Geometry check sheet. Reference: the model listing, model coordinates, mm. A direction names the side the tool comes from. Round coordinates to 2 decimals unless told otherwise and drop trailing zeros. Write each loop counter-clockwise with the first axis right and the second up, starting at its lowest first coordinate (ties: lowest second). Pieces come first, ordered by that corner, then holes. Notation, with made-up numbers: M 33,13.25 L 47,13.25 A21 cw 47,47.25 Z; hole C 20,76.5 d7. An arc over 180 degrees is marked long. Use a Markdown table: item, result.
```python
from build123d import *

# Parameters (mm, degrees)
SKETCH1_R               = 1.5
BOSS_EXTRUDE1_DEPTH     = 3.175
CUT_EXTRUDE1_DEPTH      = 131.960225355
CUT_EXTRUDE1_DEPTH_BACK = 131.960225355
SKETCH2_R               = 1.5
CUT_EXTRUDE2_DEPTH      = 131.960225355
CUT_EXTRUDE2_DEPTH_BACK = 131.960225355
SKETCH3_R               = 1.5
CUT_EXTRUDE4_DEPTH      = 40
SKETCH6_R               = 1.6
CUT_EXTRUDE5_DEPTH      = 10


with BuildPart() as part:
    # Sketch1 → Boss-Extrude1 (new body)
    with BuildSketch(Plane(origin=(0, 0, 0), x_dir=(1, 0, 0), z_dir=(0, 1, 0))):
        with BuildLine():
            Line((-10.5, 0), (-10.5, -120))
            ThreePointArc((-10.5, -120), (0, -130.5), (10.5, -120))
            Line((10.5, -120), (10.5, 0))
            ThreePointArc((10.5, 0), (0, 10.5), (-10.5, 0))
        make_face()
        with Locations(Location((0, 0, 0), (0, 0, 270))):
            Circle(SKETCH1_R, mode=Mode.SUBTRACT)
        with Locations(Location((0, -120, 0), (0, 0, 270))):
            Circle(SKETCH1_R, mode=Mode.SUBTRACT)
    extrude(amount=BOSS_EXTRUDE1_DEPTH)

    # Sketch2 → Cut-Extrude1 (cut, two sides: drawn at the far end of the back side and taken through both)
    with BuildSketch(Plane.XZ.offset(-CUT_EXTRUDE1_DEPTH_BACK)):
        with Locations(Location((0, 20, 0), (0, 0, 270))):
            Circle(SKETCH2_R)
    extrude(amount=CUT_EXTRUDE1_DEPTH + CUT_EXTRUDE1_DEPTH_BACK, mode=Mode.SUBTRACT)

    # Sketch3 → Cut-Extrude2 (cut, two sides: drawn at the far end of the back side and taken through both)
    with BuildSketch(Plane(origin=(0, 3.175, 0), x_dir=(1, 0, 0), z_dir=(0, 1, 0)).offset(-CUT_EXTRUDE2_DEPTH_BACK)):
        with Locations(Location((0, -100, 0), (0, 0, 270))):
            Circle(SKETCH3_R)
    extrude(amount=CUT_EXTRUDE2_DEPTH + CUT_EXTRUDE2_DEPTH_BACK, mode=Mode.SUBTRACT)

    # Sketch5 → Cut-Extrude4 (cut)
    with BuildSketch(Plane.XZ):
        with BuildLine():
            Line((-8.5, 10), (-8.5, 50))
            ThreePointArc((-8.5, 50), (-7.5, 51), (-6.5, 50))
            Line((-6.5, 50), (-6.5, 10))
            ThreePointArc((-6.5, 10), (-7.5, 9), (-8.5, 10))
        make_face()
        with BuildLine():
            Line((6.5, 50), (6.5, 10))
            ThreePointArc((6.5, 10), (7.5, 9), (8.5, 10))
            Line((8.5, 10), (8.5, 50))
            ThreePointArc((8.5, 50), (7.5, 51), (6.5, 50))
        make_face()
        with BuildLine():
            Line((8.5, 110), (8.5, 70))
            ThreePointArc((8.5, 70), (7.5, 69), (6.5, 70))
            Line((6.5, 70), (6.5, 110))
            ThreePointArc((6.5, 110), (7.5, 111), (8.5, 110))
        make_face()
        with BuildLine():
            Line((-6.5, 70), (-6.5, 110))
            ThreePointArc((-6.5, 110), (-7.5, 111), (-8.5, 110))
            Line((-8.5, 110), (-8.5, 70))
            ThreePointArc((-8.5, 70), (-7.5, 69), (-6.5, 70))
        make_face()
    extrude(amount=-CUT_EXTRUDE4_DEPTH, mode=Mode.SUBTRACT)

    # Sketch6 → Cut-Extrude5 (cut)
    with BuildSketch(Plane.XZ):
        with Locations(Location((0, 70.85, 0), (0, 0, 270))):
            Circle(SKETCH6_R)
        with Locations(Location((0, 32.85, 0), (0, 0, 270))):
            Circle(SKETCH6_R)
    extrude(amount=-CUT_EXTRUDE5_DEPTH, mode=Mode.SUBTRACT)


solid = part.part
```
Item 1: Cross-section at B-B, the plane y = 2. Count the separate pieces of the cut face and the enclosed holes in it, and give its area (3 significant figures).
Outcome:
| item | result |
|---|---|
| separate pieces | 1 |
| enclosed holes | 10 |
| area | 2,490 mm2 |
Item 2: Go/stop test with a flat-tipped pin: pin 1 (1 mm diameter, centred on x = -7.5, y = 2.5, fed in from +Z). Record where the tip stops, or that it passes through.
Outcome:
| item | result |
|---|---|
| pin 1 | stops at z = 127.83 |
Item 3: Cross-section at C-C, the plane z = 77.5. Record the cut outline in (x, y) (3 decimals), and give its area (3 significant figures).
Outcome:
| item | result |
|---|---|
| outline | M -10.5,0 L -8.5,0 L -8.5,3.175 L -10.5,3.175 Z; M -6.5,0 L 6.5,0 L 6.5,3.175 L -6.5,3.175 Z; M 8.5,0 L 10.5,0 L 10.5,3.175 L 8.5,3.175 Z |
| area | 54.0 mm2 |
Item 4: Access from +Z, -Z, +X, -X, +Y, -Y to the whole of each face (thin tool, end or side, straight path). Record for faces 1 (the face through (-8.5, 2, 90)), 2 (the face through (10.5, 2, 61)).
Outcome:
| item | result |
|---|---|
| face 1 | +Y, -Y |
| face 2 | +Z, -Z, +X, +Y, -Y |
Item 5: Material ranges on line 1 along X through (y, z) = (2.8, 81.5); line 2 along X through (y, z) = (1.2, 70.85); line 3 along X through (y, z) = (1.65, 120), recorded low to high. Write a range as from..to.
Outcome:
| item | result |
|---|---|
| line 1 | x = -10.5..-8.5, -6.5..6.5, 8.5..10.5 |
| line 2 | x = -10.5..-8.5, -6.5..-1.6, 1.6..6.5, 8.5..10.5 |
| line 3 | x = -10.5..-1.5, 1.5..10.5 |
Item 6: Cross-section at A-A, the plane z = 32.85. Record the cut outline in (x, y) (3 decimals).
Outcome:
| item | result |
|---|---|
| outline | M -10.5,0 L -8.5,0 L -8.5,3.175 L -10.5,3.175 Z; M -6.5,0 L -1.6,0 L -1.6,3.175 L -6.5,3.175 Z; M 1.6,0 L 6.5,0 L 6.5,3.175 L 1.6,3.175 Z; M 8.5,0 L 10.5,0 L 10.5,3.175 L 8.5,3.175 Z |
Item 7: Mould release check, pull along X, two halves, no side actions. Record for faces 3 (the face through (-0.2, 1.6, 130.5)), 4 (the face through (0, 0, 59)), 5 (the face through (6.5, 2, 90)): +X half, -X half, draft (parallel to the pull), parting line (faces both ways), or undercut.
Outcome:
| item | result |
|---|---|
| face 3 | parting line |
| face 4 | draft |
| face 5 | undercut |
